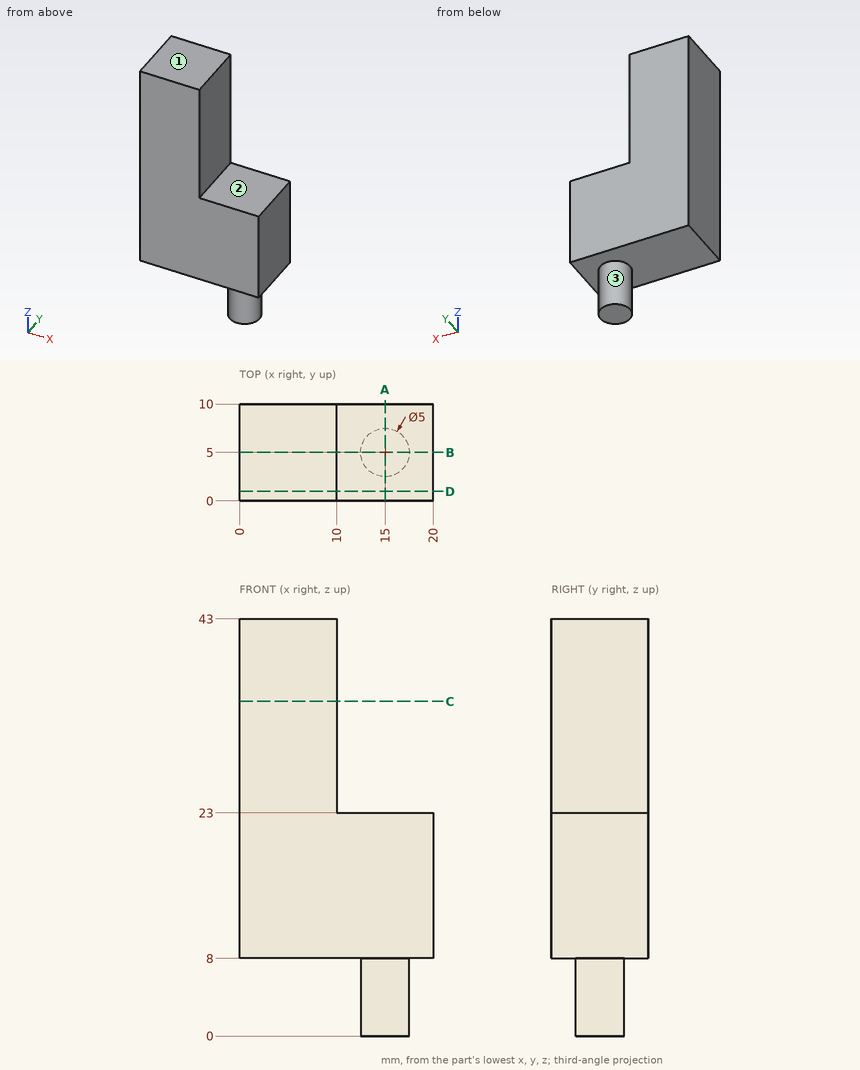
Can you work these out from the drawing? Everything is in mm from the part's minimum corner. A direction names the side the tool comes from. Give positions to 0.01 mm unless a question says otherwise; leave off trailing zeros. Loops run counter-clockwise (first coordinate to the right, second up) from the corner with the lowest first, then second, coordinate; pieces in that order, holes last. Notation, with made-up numbers: M 0,86.5 L 6,86.5 A17 ccw 6,103.5 Z; hole C -13,27 d9. An arc over 180 degrees is marked long. Use CSV: the item, a comma, the result in double quotes. Start each with the question number.
1. Imagine slicing it at D-D, the plane y = 1. Write out the boundary of the cut face in (x, z), plus the area to 3 significant figures.
2. If I drill on L1, parallel to X at y = 2.25, z = 27.5; L2, parallel to Z at x = 11.25, y = 8.25; L3, parallel to Z at x = 4.25, y = 3, over which ranges is the centre line in solid material (lowest first)?
3. Imagine slicing it at B-B, the plane y = 5. Write out the boundary of the cut face in (x, z), plus the area to 3 significant figures.
4. Imagine slicing it at C-C, the plane z = 34.5. Write out the boundary of the cut face in (x, y).
5. On a 3-axis mill with a long thin cutter (end or side, diameter ignored), from which of +Z, -Z, +X, -X, +Y, -Y can I reach the whole of each face in a straight line? I mean the marked faces 1, 2 and 3. Say none if no direction works.
6. For P1, Ø2, axis at y = 5, z = 33, coming from the +X side; P2, Ø6, axis at x = 7, z = 12, coming from the -Y side; P3, Ø6, axis at x = 8.5, y = 6, coming from the -Z side, each with a flat end and sliding along its axis, tell me the tip position at first contact or that it passes through.
7. Imagine slicing it at A-A, the plane x = 15. Write out the boundary of the cut face in (y, z), plus the area to 3 significant figures.
Response values:
1,outline,"M 0,8 L 20,8 L 20,23 L 10,23 L 10,43 L 0,43 Z"
1,area,"500 mm^2"
2,L1,"0 to 10"
2,L2,"8 to 23"
2,L3,"8 to 43"
3,outline,"M 0,8 L 12.5,8 L 12.5,0 L 17.5,0 L 17.5,8 L 20,8 L 20,23 L 10,23 L 10,43 L 0,43 Z"
3,area,"540 mm^2"
4,outline,"M 0,0 L 10,0 L 10,10 L 0,10 Z"
5,face 1,"+Z, +X, -X, +Y, -Y"
5,face 2,"+Z, +X, +Y, -Y"
5,face 3,"-Z"
6,P1,"x = 10"
6,P2,"y = 0"
6,P3,"z = 8"
7,outline,"M 0,8 L 2.5,8 L 2.5,0 L 7.5,0 L 7.5,8 L 10,8 L 10,23 L 0,23 Z"
7,area,"190 mm^2"
